Verification items for this drawing (mm, ordinates from the low corner). Round coordinates to 2 decimals unless told otherwise and drop trailing zeros. Order: outer loops, then holes, each group sorted by start corner. A loop starts at its lowest first (then second) coordinate and runs counter-clockwise, first axis right, second up. Notation, with made-up numbers: M 79.5,1.25 L 91.5,1.25 A22 cw 91.5,15.25 Z; hole C -2.5,-5.5 d8. An arc over 180 degrees is marked long. One line per item, written item: value. Start each with the question number.
(1) Cross-section at B-B, the plane y = 4. Enter the section's corners in (x, z), and give its area (3 significant figures).
(2) Release check for a two-part mould opening along X. For the marked faces 1, 2 and 3 record: released by +X, released by -X, zero draft, split by the parting line, or undercut.
(3) Depth check by flat-ended pin: pin 1 Ø2 at (x, z) = (3.5, 2.5) entering from -Y; pin 2 Ø2.5 at (x, y) = (6, 20) entering from +Z. Enter the tip coordinate at first touch or a pass-through.
(4) Cross-section at C-C, the plane z = 6.5. Enter the section's corners in (x, y), and give its area (3 significant figures).
(5) Cross-section at A-A, the plane x = 6. Enter the section's corners in (y, z), and give its area (3 significant figures).
(6) Cross-section at D-D, the plane z = 0.75. Enter the section's corners in (x, y), and give its area (3 significant figures).
(7) Thickness scan on L1, parallel to Y at x = 6, z = 3.75; L2, parallel to X at y = 4, z = 1.5; L3, parallel to Y at x = 6, z = 6. Record the ranges inside material, lowest first.
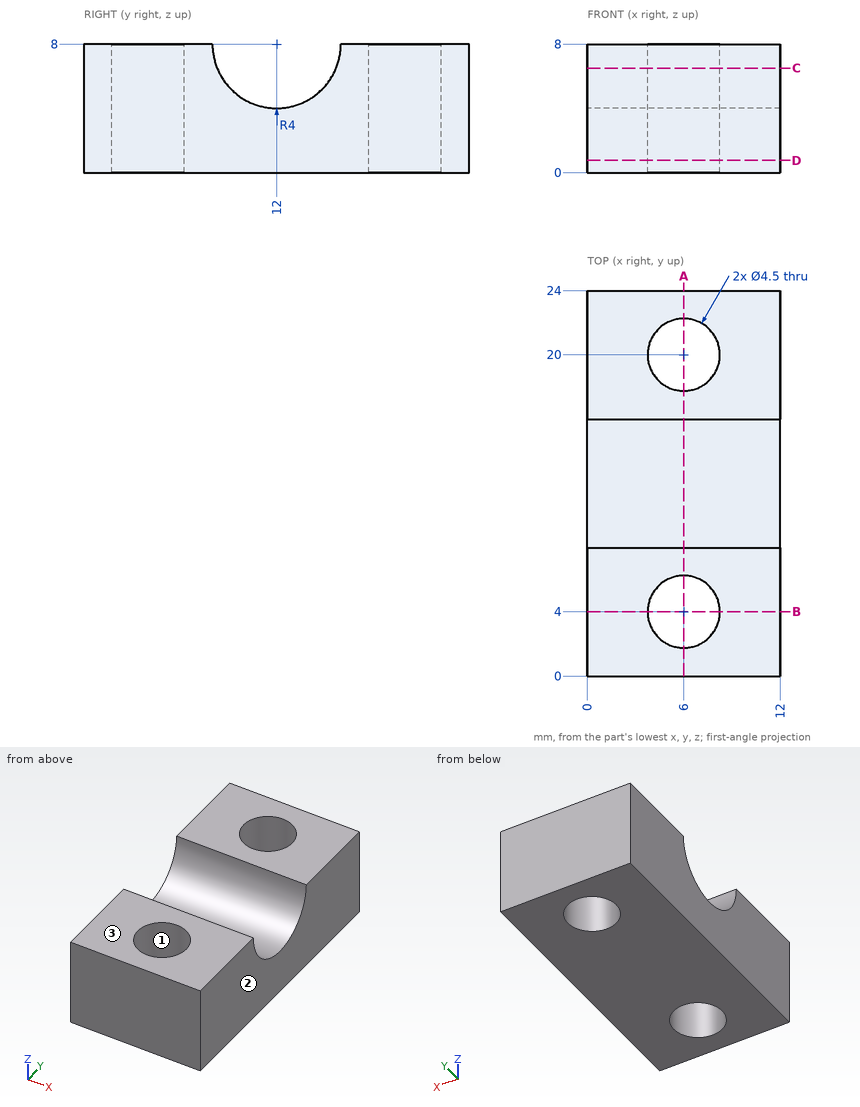
Values found:
1. outline: M 0,0 L 3.75,0 L 3.75,8 L 0,8 Z; M 8.25,0 L 12,0 L 12,8 L 8.25,8 Z
1. area: 60.0 mm^2
2. face 1: undercut
2. face 2: released by +X
2. face 3: zero draft
3. pin 1: y = 0
3. pin 2: through
4. outline: M 0,0 L 12,0 L 12,8.29 L 0,8.29 Z; M 0,15.71 L 12,15.71 L 12,24 L 0,24 Z; hole C 6,4 d4.5; hole C 6,20 d4.5
4. area: 167 mm^2
5. outline: M 0,0 L 1.75,0 L 1.75,8 L 0,8 Z; M 6.25,0 L 17.75,0 L 17.75,8 L 16,8 A4 cw 8,8 L 6.25,8 Z; M 22.25,0 L 24,0 L 24,8 L 22.25,8 Z
5. area: 94.9 mm^2
6. outline: M 0,0 L 12,0 L 12,24 L 0,24 Z; hole C 6,4 d4.5; hole C 6,20 d4.5
6. area: 256 mm^2
7. L1: 0 to 1.75, 6.25 to 17.75, 22.25 to 24
7. L2: 0 to 3.75, 8.25 to 12
7. L3: 0 to 1.75, 6.25 to 8.54, 15.46 to 17.75, 22.25 to 24
